The figure shows three views and two pictorial views of one solid part (mm, origin at its lowest corner). Answer the questions. A direction names the side the tool comes from. Coordinates: 2 decimals unless noted, no trailing zeros. Write each loop counter-clockwise with the first axis right and the second up, starting at its lowest first coordinate (ties: lowest second). Pieces come first, ordered by that corner, then holes. Notation, with made-up numbers: (-31, 14.5) - (18, 14.5) arc R6 cw to (18, 24.5) - close; hole circle Ø8 at (47, 43). An arc over 180 degrees is marked (long way). Use a Markdown table: item, result. Add a question column.
(1) The part is cut by section B-B, the plane z = 39.5. Give the vertices of the cut face in (x, y), then the cut area to 3 significant figures.
(2) For a pull along Z with two mould halves and no side action, classify the marked faces 1, 2, 3 and 4 as released by +Z, released by -Z, zero draft, split by the parting line, or undercut.
(3) A tool of negligible diameter and unlimited length cuts with its end or side. For the marked faces 5, 6 and 7, from which of +Z, -Z, +X, -X, +Y, -Y can it reach the whole face along a straight path? Write none if from no direction.
(4) The part is cut by section A-A, the plane y = 8.75. Give the vertices of the cut face in (x, z) (1 decimal), then the cut area to 3 significant figures.
(5) The part is cut by section D-D, the plane y = 11.75. Give the vertices of the cut face in (x, z) (1 decimal).
(6) The part is cut by section C-C, the plane x = 41.75. Give the vertices of the cut face in (y, z) (1 decimal).
(7) Find the intervals of material crossed by line 1 (Z direction, x = 4.5, y = 26.25) (1 decimal); line 2 (Y direction, x = 46, z = 27.5); line 3 (Z direction, x = 8.5, y = 6) (1 decimal), in increasing order. Write a range as from..to.
(8) Given pin 1 Ø5 at (x, z) = (36.5, 42) entering from +Y; pin 2 Ø1.5 at (y, z) = (14.5, 40.5) entering from +X; pin 3 Ø3 at (x, y) = (5.5, 19.5) entering from +Z, each flat-ended and moving along its own axis, determine where each tip first touches the part or whether it passes through.
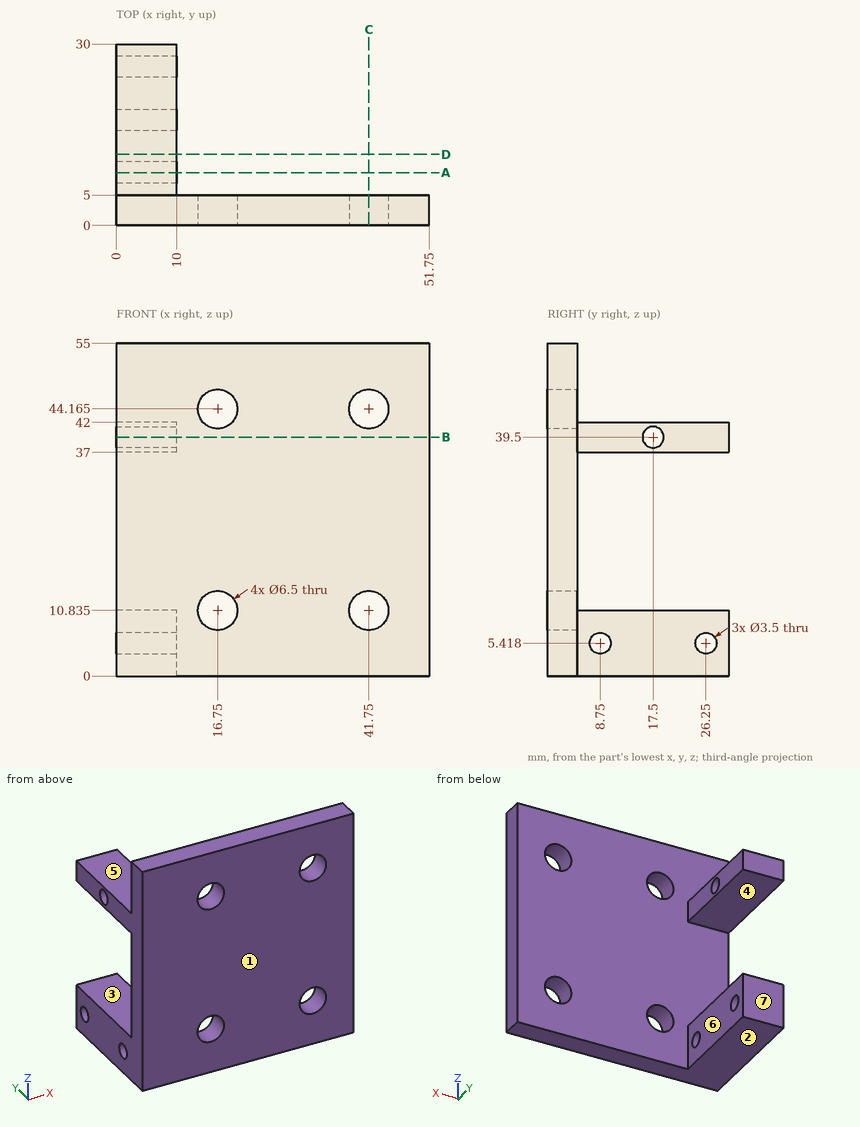
Model answer:
| question | item | result |
|---|---|---|
| 1 | outline | (0, 0) - (51.75, 0) - (51.75, 5) - (10, 5) - (10, 15.75) - (0, 15.75) - close; (0, 19.25) - (10, 19.25) - (10, 30) - (0, 30) - close |
| 1 | area | 474 mm^2 |
| 2 | face 1 | zero draft |
| 2 | face 2 | released by -Z |
| 2 | face 3 | undercut |
| 2 | face 4 | undercut |
| 3 | face 5 | +Z, +X, -X, +Y |
| 3 | face 6 | +Z, -Z, +X, +Y |
| 3 | face 7 | +Z, -Z, +X, -X, +Y |
| 4 | outline | (0, 0) - (10, 0) - (10, 3.7) - (0, 3.7) - close; (0, 7.2) - (10, 7.2) - (10, 10.8) - (0, 10.8) - close; (0, 37) - (10, 37) - (10, 42) - (0, 42) - close |
| 4 | area | 123 mm^2 |
| 5 | outline | (0, 0) - (10, 0) - (10, 10.8) - (0, 10.8) - close; (0, 37) - (10, 37) - (10, 42) - (0, 42) - close |
| 6 | outline | (0, 0) - (5, 0) - (5, 7.6) - (0, 7.6) - close; (0, 14.1) - (5, 14.1) - (5, 40.9) - (0, 40.9) - close; (0, 47.4) - (5, 47.4) - (5, 55) - (0, 55) - close |
| 7 | line 1 | 0..3.7, 7.2..10.8, 37..42 |
| 7 | line 2 | 0..5 |
| 7 | line 3 | 0..10.8, 37..42 |
| 8 | pin 1 | y = 5 |
| 8 | pin 2 | x = 10 |
| 8 | pin 3 | z = 42 |
